Geometry check sheet. Reference: the model listing, model coordinates, mm. A direction names the side the tool comes from. Give positions to 0.01 mm unless a question says otherwise; leave off trailing zeros. Loops run counter-clockwise (first coordinate to the right, second up) from the corner with the lowest first, then second, coordinate; pieces in that order, holes last. Notation, with made-up numbers: (9, 70) - (30, 70) arc R31 cw to (30, 94) - close; hole circle Ø1 at (84.5, -34.75). An arc over 180 degrees is marked (long way). Use a Markdown table: item, result. Add a question column.
1. Draft check along Z on faces 5 (the flat face through (10, -10, -5)), 6 (the cylindrical face through (11.675, -2.958, -7.536)), 7 (the flat face through (-15.5, -3, 0)). Enter one of: pulls with the +Z half, pulls with the -Z half, needs draft (parallel to the pull), parting line crosses it, or undercut.
2. Material ranges on L1, parallel to X at y = -4.4, z = -9; L2, parallel to Z at x = 12, y = -4.5; L3, parallel to X at y = -4.5, z = -8.5, recorded low to high.
3. Set-up check for faces 1 (the flat face through (1.73, -16.39, 0.17)), 2 (the flat face through (-11, -11, 5)), 3 (the flat face through (10, -10, 5)), 4 (the flat face through (8.438, -13, -8)): record each of +Z, -Z, +X, -X, +Y, -Y from which the full face is reachable in a straight line by a thin tool's end or side.
4. Cross-section at C-C on x = 12. Enter the section's corners in (y, z).
5. Depth check by flat-ended pin: P1, Ø1.8, axis at x = 10.5, y = -14, coming from the -Z side; P2, Ø3, axis at x = -3.5, z = 8.5, coming from the +Y side; P3, Ø2, axis at x = 12.5, z = -5.5, coming from the -Y side; P4, Ø2.5, axis at x = -12, z = -9, coming from the +Y side. Enter the tip coordinate at first touch or a pass-through.
6. Cross-section at D-D on y = -14.5. Enter the section's corners in (x, z), and give its area (3 significant figures).
7. Cross-section at B-B on z = -9. Enter the section's corners in (x, y), and give its area (3 significant figures).
8. Cross-section at A-A on y = -2.5. Enter the section's corners in (x, z).
from build123d import *

# Parameters (mm, degrees)
SALIENTE_EXTRUIR2_DEPTH = 12
SALIENTE_EXTRUIR3_DEPTH = 5
CORTAR_EXTRUIR1_REACH   = 21
CROQUIS4_R              = 1.5


with BuildPart() as part:
    # Croquis2 → Saliente-Extruir2 (new body, symmetric)
    with BuildSketch(Plane.XY):
        with BuildLine():
            Line((8.438000444, -19), (8.438000444, -6))
            Line((8.438000444, -6), (14.5, -6))
            Line((14.5, -6), (15.5, -6))
            Line((15.5, -6), (15.5, 0))
            Line((15.5, 0), (-15.5, 0))
            Line((-15.5, 0), (-15.5, -6))
            Line((-15.5, -6), (-14.5, -6))
            Line((-14.5, -6), (-8.438000444, -6))
            Line((-8.438000444, -6), (-8.438000444, -19))
            Line((-8.438000444, -19), (-2.438000444, -19))
            Line((-2.438000444, -19), (-1.045861913, -13.860851313))
            ThreePointArc((-1.045861913, -13.860851313), (-2.430694587, -6.823252634), (4, -10))
            ThreePointArc((4, -10), (3.176747366, -12.430694587), (1.045861913, -13.860851313))
            Line((1.045861913, -13.860851313), (2.438000444, -19))
            Line((2.438000444, -19), (8.438000444, -19))
        make_face()
    extrude(amount=SALIENTE_EXTRUIR2_DEPTH, both=True)

    # Croquis3 → Saliente-Extruir3 (add, symmetric)
    with BuildSketch(Plane.XY):
        Polygon((8.438000444, -6), (14.5, -6), (8.438000444, -19), align=None)
        Polygon((-8.438000444, -6), (-8.438000444, -19), (-14.5, -6), align=None)
    extrude(amount=SALIENTE_EXTRUIR3_DEPTH, both=True)

    # Croquis4 → Cortar-Extruir1 (cut, up to next)
    with BuildSketch(Plane(origin=(0, 0, 0), x_dir=(1, 0, 0), z_dir=(0, 1, 0)), mode=Mode.PRIVATE) as cortar_extruir1_sk1:
        with Locations((-12, 9)):
            Circle(CROQUIS4_R)
    cortar_extruir1_tool1 = extrude(cortar_extruir1_sk1.sketch, amount=-CORTAR_EXTRUIR1_REACH, mode=Mode.PRIVATE) & part.part
    add(cortar_extruir1_tool1.solids().sort_by_distance((-12, 0, -9))[0], mode=Mode.SUBTRACT)
    # Croquis4 → Cortar-Extruir1 (cut, up to next)
    with BuildSketch(Plane(origin=(0, 0, 0), x_dir=(1, 0, 0), z_dir=(0, 1, 0)), mode=Mode.PRIVATE) as cortar_extruir1_sk2:
        with Locations((12, 9)):
            Circle(CROQUIS4_R)
    cortar_extruir1_tool2 = extrude(cortar_extruir1_sk2.sketch, amount=-CORTAR_EXTRUIR1_REACH, mode=Mode.PRIVATE) & part.part
    add(cortar_extruir1_tool2.solids().sort_by_distance((12, 0, -9))[0], mode=Mode.SUBTRACT)
    # Croquis4 → Cortar-Extruir1 (cut, up to next)
    with BuildSketch(Plane(origin=(0, 0, 0), x_dir=(1, 0, 0), z_dir=(0, 1, 0)), mode=Mode.PRIVATE) as cortar_extruir1_sk3:
        with Locations((12, -9)):
            Circle(CROQUIS4_R)
    cortar_extruir1_tool3 = extrude(cortar_extruir1_sk3.sketch, amount=-CORTAR_EXTRUIR1_REACH, mode=Mode.PRIVATE) & part.part
    add(cortar_extruir1_tool3.solids().sort_by_distance((12, 0, 9))[0], mode=Mode.SUBTRACT)
    # Croquis4 → Cortar-Extruir1 (cut, up to next)
    with BuildSketch(Plane(origin=(0, 0, 0), x_dir=(1, 0, 0), z_dir=(0, 1, 0)), mode=Mode.PRIVATE) as cortar_extruir1_sk4:
        with Locations((-12, -9)):
            Circle(CROQUIS4_R)
    cortar_extruir1_tool4 = extrude(cortar_extruir1_sk4.sketch, amount=-CORTAR_EXTRUIR1_REACH, mode=Mode.PRIVATE) & part.part
    add(cortar_extruir1_tool4.solids().sort_by_distance((-12, 0, 9))[0], mode=Mode.SUBTRACT)


solid = part.part
Values found:
| question | item | result |
|---|---|---|
| 1 | face 5 | pulls with the -Z half |
| 1 | face 6 | undercut |
| 1 | face 7 | needs draft |
| 2 | L1 | x = -15.5 to -13.5, -10.5 to 10.5, 13.5 to 15.5 |
| 2 | L2 | z = -12 to -10.5, -7.5 to 7.5, 10.5 to 12 |
| 2 | L3 | x = -15.5 to -13.41, -10.59 to 10.59, 13.41 to 15.5 |
| 3 | face 1 | +Z, -Z, -Y |
| 3 | face 2 | +Z, -X, -Y |
| 3 | face 3 | +Z, +X, -Y |
| 3 | face 4 | -Z, +X, -Y |
| 4 | outline | (-11.36, -5) - (-6, -5) - (-6, -7.5) - (0, -7.5) - (0, 7.5) - (-6, 7.5) - (-6, 5) - (-11.36, 5) - close; (-6, -12) - (0, -12) - (0, -10.5) - (-6, -10.5) - close; (-6, 10.5) - (0, 10.5) - (0, 12) - (-6, 12) - close |
| 5 | P1 | stops at z = -5 |
| 5 | P2 | stops at y = 0 |
| 5 | P3 | stops at y = -12.15 |
| 5 | P4 | passes through |
| 6 | outline | (-10.54, -5) - (-8.44, -5) - (-8.44, -12) - (-1.22, -12) - (-1.22, 12) - (-8.44, 12) - (-8.44, 5) - (-10.54, 5) - close; (1.22, -12) - (8.44, -12) - (8.44, -5) - (10.54, -5) - (10.54, 5) - (8.44, 5) - (8.44, 12) - (1.22, 12) - close |
| 6 | area | 388 mm2 |
| 7 | outline | (-15.5, -6) - (-13.5, -6) - (-13.5, 0) - (-15.5, 0) - close; (-10.5, -6) - (-8.44, -6) - (-8.44, -19) - (-2.44, -19) - (-1.05, -13.86) arc R4 cw (long way) to (1.05, -13.86) - (2.44, -19) - (8.44, -19) - (8.44, -6) - (10.5, -6) - (10.5, 0) - (-10.5, 0) - close; (13.5, -6) - (15.5, -6) - (15.5, 0) - (13.5, 0) - close |
| 7 | area | 301 mm2 |
| 8 | outline | (-15.5, -12) - (15.5, -12) - (15.5, 12) - (-15.5, 12) - close; hole circle Ø3 at (-12, -9); hole circle Ø3 at (-12, 9); hole circle Ø3 at (12, -9); hole circle Ø3 at (12, 9) |
